Build history of the part. All positions in model axes, mm. Face numbers are marked on the shaded views. Round coordinates to 2 decimals unless told otherwise and drop trailing zeros. Write each loop counter-clockwise with the first axis right and the second up, starting at its lowest first coordinate (ties: lowest second). Pieces come first, ordered by that corner, then holes. Notation, with made-up numbers: (78, -33) -> (118, -33) arc R3 cw to (118, -29) -> close; hole circle Ø3 at (-26, 33.5). An arc over 180 degrees is marked (long way). Return JSON: item names as keys, results as strings.
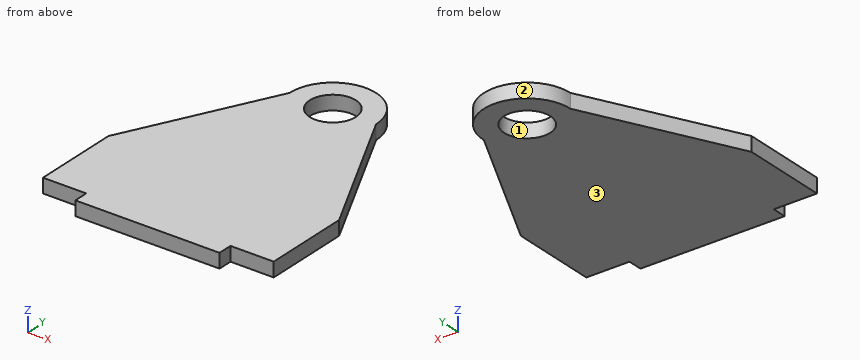
from build123d import *

# Parameters (mm, degrees)
SKETCH1_R           = 8
BOSS_EXTRUDE1_DEPTH = 5


with BuildPart() as part:
    # Sketch1 → Boss-Extrude1 (new body)
    with BuildSketch(Plane.XY):
        with BuildLine():
            Line((-40, -80), (-25, -80))
            Line((-25, -80), (-25, -85))
            Line((-25, -85), (25, -85))
            Line((25, -85), (25, -80))
            Line((25, -80), (40, -80))
            Line((40, -80), (40, -50))
            Line((40, -50), (15, 0))
            ThreePointArc((15, 0), (0, 15), (-15, 0))
            Line((-15, 0), (-40, -50))
            Line((-40, -50), (-40, -80))
        make_face()
        Circle(SKETCH1_R, mode=Mode.SUBTRACT)
    extrude(amount=BOSS_EXTRUDE1_DEPTH)


solid = part.part
Q1. Saw through at A-A on x = 0. List the corners of the cut face in (y, z), then the cut area to 3 significant figures.
Verdict:
{"outline": "(-85, 0) -> (-8, 0) -> (-8, 5) -> (-85, 5) -> close; (8, 0) -> (15, 0) -> (15, 5) -> (8, 5) -> close", "area": "420 mm²"}
Q2. Two-plate mould, pull along Y, no slides. Class the marked faces 1, 2 and 3: +Y half, -Y half, draft (parallel to the pull), parting line (faces both ways), or undercut.
Verdict:
{"face 1": "undercut", "face 2": "+Y half", "face 3": "draft"}
Q3. Pin check, flat tips, straight feed: pin 1 Ø1.5 at (y, z) = (-83.5, 3) entering from -X; pin 2 Ø3 at (x, z) = (-20.5, 0.5) entering from +Y; pin 3 Ø13 at (x, y) = (0, 0) entering from -Z; pin 4 Ø2 at (x, z) = (-25, 2) entering from +Y. Stop position of each tip, or through.
Verdict:
{"pin 1": "stops at x = -25", "pin 2": "stops at y = -8", "pin 3": "passes through", "pin 4": "stops at y = -18"}
Q4. Saw through at C-C on y = -4. List the corners of the cut face in (x, z), then the cut area to 3 significant figures.
Verdict:
{"outline": "(-17, 0) -> (-6.93, 0) -> (-6.93, 5) -> (-17, 5) -> close; (6.93, 0) -> (17, 0) -> (17, 5) -> (6.93, 5) -> close", "area": "101 mm²"}
Q5. Saw through at D-D on x = 18. List the corners of the cut face in (y, z), then the cut area to 3 significant figures.
Verdict:
{"outline": "(-85, 0) -> (-6, 0) -> (-6, 5) -> (-85, 5) -> close", "area": "395 mm²"}
Q6. Saw through at B-B on z = 1.95. List the corners of the cut face in (x, y).
Verdict:
{"outline": "(-40, -80) -> (-25, -80) -> (-25, -85) -> (25, -85) -> (25, -80) -> (40, -80) -> (40, -50) -> (15, 0) arc R15 ccw to (-15, 0) -> (-40, -50) -> close; hole circle Ø16 at (0, 0)"}
Q7. Wall check: L1, parallel to Y at x = 0, z = 3.45; L2, parallel to Y at x = -6, z = 3; L3, parallel to Y at x = -19, z = 3.35. Give the ranges that are in metal, low to high.
Verdict:
{"L1": "y = -85 to -8, 8 to 15", "L2": "y = -85 to -5.29, 5.29 to 13.75", "L3": "y = -85 to -8"}
